Source: CAD feature listing. Evaluate the final solid. Frame: model axes, mm. Give positions to 0.01 mm unless a question says otherwise; leave off trailing zeros. Order: outer loops, then holes, each group sorted by start corner. A loop starts at its lowest first (then second) coordinate and runs counter-clockwise, first axis right, second up. Notation, with made-up numbers: M -33.5,-1.75 L 16.5,-1.75 A25 ccw 16.5,28.25 Z; hole C 49.5,60.5 d7. An arc over 180 degrees is marked long. Return JSON: item names as keys, results as strings.
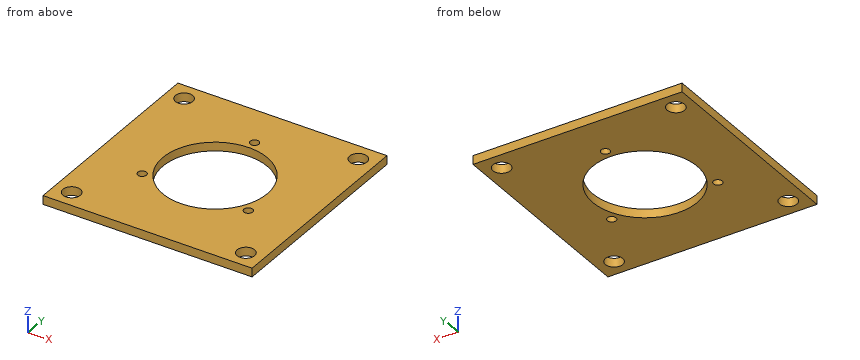
Autodesk Inventor part; units mm, degrees
ref_plane "YZ Plane" through (0, 0, 0) normal (1, 0, 0) x (0, 1, 0)
ref_plane "XZ Plane" through (0, 0, 0) normal (0, 1, 0) x (-1, 0, 0)
ref_plane "XY Plane" through (0, 0, 0) normal (0, 0, 1) x (1, 0, 0)
sketch "Sketch1" plane through (0, 0, 0) normal (0, 0, 1) x (1, 0, 0)
  line L0 (-38.1, 38.1) -> (38.1, 38.1)
  line L1 (38.1, 38.1) -> (38.1, -38.1)
  line L2 (38.1, -38.1) -> (-38.1, -38.1)
  line L3 (-38.1, -38.1) -> (-38.1, 38.1)
  circle A0 centre (0, 0) radius 19.05
  point P0 (-31.75, 31.75)
  point P1 (31.75, 31.75)
  point P2 (31.75, -31.75)
  point P3 (-31.75, -31.75)
  dimension "d0" = 76.2
  dimension "d1" = 76.2
  dimension "d2" = 38.1
  dimension "d3" = 38.1
  dimension "d4" = 38.1
  dimension "d5" = 6.35
  dimension "d6" = 6.35
  dimension "d7" = 6.35
  dimension "d8" = 6.35
extrude "Extrusion1" add sketch "Sketch1" against normal blind 3.175
hole "Hole1" at (-31.75, 31.75, 0) at (31.75, 31.75, 0) at (31.75, -31.75, 0) at (-31.75, -31.75, 0) direction (0, 0, -1) diameter 6.35 end through all
sketch "Sketch2" plane through (0, 0, 0) normal (0, 0, 1) x (1, 0, 0)
  circle A0 centre (0, 0) radius 19.05
  line L0 (-38.1, 38.1) -> (38.1, 38.1)
  line L1 (-38.1, -38.1) -> (-38.1, 38.1)
  line L2 (38.1, -38.1) -> (-38.1, -38.1)
  line L3 (38.1, 38.1) -> (38.1, -38.1)
  circle A1 centre (0, 0) radius 19.05
  circle A2 centre (0, 0) radius 22.3343
  point P0 (0, 22.3343)
  point P1 (19.3421, -11.1672)
  point P2 (-19.3421, -11.1672)
  dimension "d19" = 38.6842
  dimension "d20" = 38.6842
  dimension "d21" = 38.6842
  dimension "d22" = 44.6687
  dimension "d24" = 38.1
hole "Hole2" at (0, 22.3343, 0) at (19.3421, -11.1672, 0) at (-19.3421, -11.1672, 0) direction (0, 0, -1) diameter 3.175 end through all
equation "\"d24\" = 0.5 * d1"
properties part number "Top Plate BD Motor mount"
1. Section query A-A (x = 0). Return loops of the section in (y, z) (3 decimals), then the cut area to 3 significant figures.
Evaluation:
{"outline": "M -38.1,-3.175 L -19.05,-3.175 L -19.05,0 L -38.1,0 Z; M 19.05,-3.175 L 20.747,-3.175 L 20.747,0 L 19.05,0 Z; M 23.922,-3.175 L 38.1,-3.175 L 38.1,0 L 23.922,0 Z", "area": "111 mm^2"}
2. Section query B-B (y = 0). Return loops of the section in (x, z) (3 decimals), then the cut area to 3 significant figures.
Evaluation:
{"outline": "M -38.1,-3.175 L -19.05,-3.175 L -19.05,0 L -38.1,0 Z; M 19.05,-3.175 L 38.1,-3.175 L 38.1,0 L 19.05,0 Z", "area": "121 mm^2"}
3. Section query C-C (y = -31.75). Return loops of the section in (x, z) (3 decimals).
Evaluation:
{"outline": "M -38.1,-3.175 L -34.925,-3.175 L -34.925,0 L -38.1,0 Z; M -28.575,-3.175 L 28.575,-3.175 L 28.575,0 L -28.575,0 Z; M 34.925,-3.175 L 38.1,-3.175 L 38.1,0 L 34.925,0 Z"}
4. Section query D-D (z = -0.5). State how many separate pieces and enclosed holes the cut face has, then the cut area to 3 significant figures.
Evaluation:
{"separate pieces": "1", "enclosed holes": "8", "area": "4,520 mm^2"}
5. First-contact query: pin 1 (3 mm diameter, centred on x = 0, y = 22.33, fed in from +Z). Flat tip, straight axial feed; report the tip coordinate or a pass-through.
Evaluation:
{"pin 1": "passes through"}
6. Ray query, probe 1 along Y at (x, z) = (31.75, -2.05) (3 decimals); probe 2 along Y at (x, z) = (0, -2.2). Return the intervals inside material, ascending.
Evaluation:
{"probe 1": "y = -38.1 to -34.925, -28.575 to 28.575, 34.925 to 38.1", "probe 2": "y = -38.1 to -19.05, 19.05 to 20.75, 23.92 to 38.1"}
